Here's how the part is built. I have some questions about the finished solid (model axes, mm). Give positions to 0.01 mm unless a question says otherwise; leave off trailing zeros. Order: outer loops, then holes, each group sorted by start corner. A loop starts at its lowest first (then second) coordinate and runs counter-clockwise, first axis right, second up. Notation, with made-up numbers: M 32.5,-12.75 L 42.5,-12.75 A13 cw 42.5,12.25 Z; hole C -33.75,-1 d7. An arc over 180 degrees is marked long. One line per item, written item: value. Start each with the question number.
from build123d import *

# Parameters (mm, degrees)
SKETCH1_W           = 65.5
SKETCH1_H           = 65.5
BOSS_EXTRUDE1_DEPTH = 3
CUT_EXTRUDE1_REACH  = 48.413
SKETCH2_R           = 2.6
SKETCH2_R_2         = 3.6
FILLET1_R           = 3


with BuildPart() as part:
    # Sketch1 → Boss-Extrude1 (new body)
    with BuildSketch(Plane.XY):
        Rectangle(SKETCH1_W, SKETCH1_H)
    extrude(amount=BOSS_EXTRUDE1_DEPTH)

    # Sketch2 → Cut-Extrude1 (cut, up to next)
    with BuildSketch(Plane.XY.offset(3), mode=Mode.PRIVATE) as cut_extrude1_sk1:
        Circle(SKETCH2_R)
    cut_extrude1_tool1 = extrude(cut_extrude1_sk1.sketch, amount=-CUT_EXTRUDE1_REACH, mode=Mode.PRIVATE) & part.part
    # Sketch2 → Cut-Extrude1 (cut, up to next)
    with BuildSketch(Plane.XY.offset(3), mode=Mode.PRIVATE) as cut_extrude1_sk2:
        with Locations((10, 0)):
            Circle(SKETCH2_R)
    cut_extrude1_tool2 = extrude(cut_extrude1_sk2.sketch, amount=-CUT_EXTRUDE1_REACH, mode=Mode.PRIVATE) & part.part
    # Sketch2 → Cut-Extrude1 (cut, up to next)
    with BuildSketch(Plane.XY.offset(3), mode=Mode.PRIVATE) as cut_extrude1_sk3:
        with Locations((20, 0)):
            Circle(SKETCH2_R)
    cut_extrude1_tool3 = extrude(cut_extrude1_sk3.sketch, amount=-CUT_EXTRUDE1_REACH, mode=Mode.PRIVATE) & part.part
    # Sketch2 → Cut-Extrude1 (cut, up to next)
    with BuildSketch(Plane.XY.offset(3), mode=Mode.PRIVATE) as cut_extrude1_sk4:
        with Locations((0, -10)):
            Circle(SKETCH2_R)
    cut_extrude1_tool4 = extrude(cut_extrude1_sk4.sketch, amount=-CUT_EXTRUDE1_REACH, mode=Mode.PRIVATE) & part.part
    # Sketch2 → Cut-Extrude1 (cut, up to next)
    with BuildSketch(Plane.XY.offset(3), mode=Mode.PRIVATE) as cut_extrude1_sk5:
        with Locations((20, -10)):
            Circle(SKETCH2_R)
    cut_extrude1_tool5 = extrude(cut_extrude1_sk5.sketch, amount=-CUT_EXTRUDE1_REACH, mode=Mode.PRIVATE) & part.part
    # Sketch2 → Cut-Extrude1 (cut, up to next)
    with BuildSketch(Plane.XY.offset(3), mode=Mode.PRIVATE) as cut_extrude1_sk6:
        with Locations((20, 10)):
            Circle(SKETCH2_R)
    cut_extrude1_tool6 = extrude(cut_extrude1_sk6.sketch, amount=-CUT_EXTRUDE1_REACH, mode=Mode.PRIVATE) & part.part
    # Sketch2 → Cut-Extrude1 (cut, up to next)
    with BuildSketch(Plane.XY.offset(3), mode=Mode.PRIVATE) as cut_extrude1_sk7:
        with Locations((0, 10)):
            Circle(SKETCH2_R)
    cut_extrude1_tool7 = extrude(cut_extrude1_sk7.sketch, amount=-CUT_EXTRUDE1_REACH, mode=Mode.PRIVATE) & part.part
    # Sketch2 → Cut-Extrude1 (cut, up to next)
    with BuildSketch(Plane.XY.offset(3), mode=Mode.PRIVATE) as cut_extrude1_sk8:
        with Locations((-20, -10)):
            Circle(SKETCH2_R)
    cut_extrude1_tool8 = extrude(cut_extrude1_sk8.sketch, amount=-CUT_EXTRUDE1_REACH, mode=Mode.PRIVATE) & part.part
    # Sketch2 → Cut-Extrude1 (cut, up to next)
    with BuildSketch(Plane.XY.offset(3), mode=Mode.PRIVATE) as cut_extrude1_sk9:
        with Locations((-20, 10)):
            Circle(SKETCH2_R)
    cut_extrude1_tool9 = extrude(cut_extrude1_sk9.sketch, amount=-CUT_EXTRUDE1_REACH, mode=Mode.PRIVATE) & part.part
    # Sketch2 → Cut-Extrude1 (cut, up to next)
    with BuildSketch(Plane.XY.offset(3), mode=Mode.PRIVATE) as cut_extrude1_sk10:
        with Locations((-20, 0)):
            Circle(SKETCH2_R)
    cut_extrude1_tool10 = extrude(cut_extrude1_sk10.sketch, amount=-CUT_EXTRUDE1_REACH, mode=Mode.PRIVATE) & part.part
    # Sketch2 → Cut-Extrude1 (cut, up to next)
    with BuildSketch(Plane.XY.offset(3), mode=Mode.PRIVATE) as cut_extrude1_sk11:
        with Locations((-10, 0)):
            Circle(SKETCH2_R)
    cut_extrude1_tool11 = extrude(cut_extrude1_sk11.sketch, amount=-CUT_EXTRUDE1_REACH, mode=Mode.PRIVATE) & part.part
    # Sketch2 → Cut-Extrude1 (cut, up to next)
    with BuildSketch(Plane.XY.offset(3), mode=Mode.PRIVATE) as cut_extrude1_sk12:
        with Locations((-20, 20)):
            Circle(SKETCH2_R_2)
    cut_extrude1_tool12 = extrude(cut_extrude1_sk12.sketch, amount=-CUT_EXTRUDE1_REACH, mode=Mode.PRIVATE) & part.part
    # Sketch2 → Cut-Extrude1 (cut, up to next)
    with BuildSketch(Plane.XY.offset(3), mode=Mode.PRIVATE) as cut_extrude1_sk13:
        with Locations((20, 20)):
            Circle(SKETCH2_R_2)
    cut_extrude1_tool13 = extrude(cut_extrude1_sk13.sketch, amount=-CUT_EXTRUDE1_REACH, mode=Mode.PRIVATE) & part.part
    # Sketch2 → Cut-Extrude1 (cut, up to next)
    with BuildSketch(Plane.XY.offset(3), mode=Mode.PRIVATE) as cut_extrude1_sk14:
        with Locations((20, -20)):
            Circle(SKETCH2_R_2)
    cut_extrude1_tool14 = extrude(cut_extrude1_sk14.sketch, amount=-CUT_EXTRUDE1_REACH, mode=Mode.PRIVATE) & part.part
    # Sketch2 → Cut-Extrude1 (cut, up to next)
    with BuildSketch(Plane.XY.offset(3), mode=Mode.PRIVATE) as cut_extrude1_sk15:
        with Locations((-20, -20)):
            Circle(SKETCH2_R_2)
    cut_extrude1_tool15 = extrude(cut_extrude1_sk15.sketch, amount=-CUT_EXTRUDE1_REACH, mode=Mode.PRIVATE) & part.part
    add(cut_extrude1_tool1.solids().sort_by_distance((0, 0, 3))[0], mode=Mode.SUBTRACT)
    add(cut_extrude1_tool2.solids().sort_by_distance((10, 0, 3))[0], mode=Mode.SUBTRACT)
    add(cut_extrude1_tool3.solids().sort_by_distance((20, 0, 3))[0], mode=Mode.SUBTRACT)
    add(cut_extrude1_tool4.solids().sort_by_distance((0, -10, 3))[0], mode=Mode.SUBTRACT)
    add(cut_extrude1_tool5.solids().sort_by_distance((20, -10, 3))[0], mode=Mode.SUBTRACT)
    add(cut_extrude1_tool6.solids().sort_by_distance((20, 10, 3))[0], mode=Mode.SUBTRACT)
    add(cut_extrude1_tool7.solids().sort_by_distance((0, 10, 3))[0], mode=Mode.SUBTRACT)
    add(cut_extrude1_tool8.solids().sort_by_distance((-20, -10, 3))[0], mode=Mode.SUBTRACT)
    add(cut_extrude1_tool9.solids().sort_by_distance((-20, 10, 3))[0], mode=Mode.SUBTRACT)
    add(cut_extrude1_tool10.solids().sort_by_distance((-20, 0, 3))[0], mode=Mode.SUBTRACT)
    add(cut_extrude1_tool11.solids().sort_by_distance((-10, 0, 3))[0], mode=Mode.SUBTRACT)
    add(cut_extrude1_tool12.solids().sort_by_distance((-20, 20, 3))[0], mode=Mode.SUBTRACT)
    add(cut_extrude1_tool13.solids().sort_by_distance((20, 20, 3))[0], mode=Mode.SUBTRACT)
    add(cut_extrude1_tool14.solids().sort_by_distance((20, -20, 3))[0], mode=Mode.SUBTRACT)
    add(cut_extrude1_tool15.solids().sort_by_distance((-20, -20, 3))[0], mode=Mode.SUBTRACT)

    # Fillet1
    fillet1_edges = [part.edges().sort_by_distance(p)[0] for p in [
        (-32.75, 32.75, 1.5),
        (-32.75, -32.75, 1.5),
        (32.75, -32.75, 1.5),
        (32.75, 32.75, 1.5),
    ]]
    fillet(fillet1_edges, radius=FILLET1_R)


solid = part.part
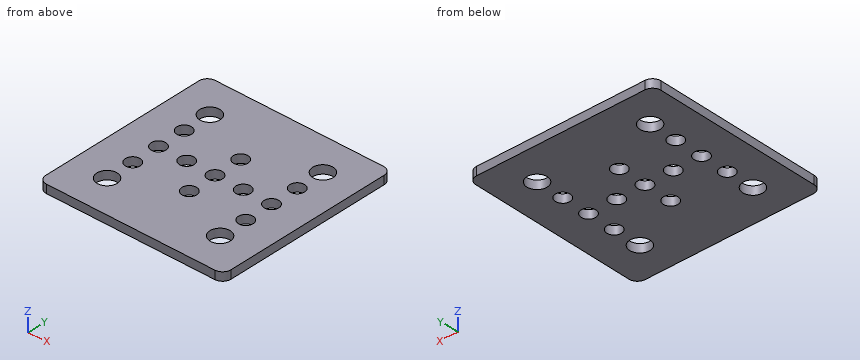
Item 1: I want a section at C-C on z = 1.4. Count the separate pieces of the cut face and the enclosed holes in it, plus the area to 3 significant figures.
Item 2: I want a section at D-D on y = -20. Write out the boundary of the cut face in (x, z).
Item 3: I want a section at A-A on x = 10. Write out the boundary of the cut face in (y, z), plus the area to 3 significant figures.
Item 4: Please list where these lines run through material, in increasing order: probe 1 along Y at (x, z) = (-20, 1.9); probe 2 along Y at (x, z) = (0, 0.85); probe 3 along X at (y, z) = (-9.5, 0.85). Write a range as [from, to].
Item 5: Will this pin go through, and if not, where does the flat tip stop? P1, Ø4.5, axis at x = 20, y = -10, coming from the +Z side.
Item 6: I want a section at B-B on y = 0. Write out the boundary of the cut face in (x, z), plus the area to 4 significant figures.
Answer below:
1. separate pieces: 1
1. enclosed holes: 15
1. area: 3,890 mm²
2. outline: M -32.75,0 L -23.6,0 L -23.6,3 L -32.75,3 Z; M -16.4,0 L 16.4,0 L 16.4,3 L -16.4,3 Z; M 23.6,0 L 32.75,0 L 32.75,3 L 23.6,3 Z
3. outline: M -32.75,0 L -2.6,0 L -2.6,3 L -32.75,3 Z; M 2.6,0 L 32.75,0 L 32.75,3 L 2.6,3 Z
3. area: 181 mm²
4. probe 1: y = [-32.75, -23.6], [-16.4, -12.6], [-7.4, -2.6], [2.6, 7.4], [12.6, 16.4], [23.6, 32.75]
4. probe 2: y = [-32.75, -12.6], [-7.4, -2.6], [2.6, 7.4], [12.6, 32.75]
4. probe 3: x = [-32.75, -22.55], [-17.45, -2.55], [2.55, 17.45], [22.55, 32.75]
5. P1: passes through
6. outline: M -32.75,0 L -22.6,0 L -22.6,3 L -32.75,3 Z; M -17.4,0 L -12.6,0 L -12.6,3 L -17.4,3 Z; M -7.4,0 L -2.6,0 L -2.6,3 L -7.4,3 Z; M 2.6,0 L 7.4,0 L 7.4,3 L 2.6,3 Z; M 12.6,0 L 17.4,0 L 17.4,3 L 12.6,3 Z; M 22.6,0 L 32.75,0 L 32.75,3 L 22.6,3 Z
6. area: 118.5 mm²
